Geometry: final body of the model. Coordinates: model frame, mm. Face numbers are marked on the shaded views. Give positions to 0.01 mm unless a question says otherwise; leave off trailing zeros. Write each loop counter-clockwise with the first axis right and the second up, starting at its lowest first coordinate (ties: lowest second). Pieces come first, ordered by that corner, then holes. Notation, with made-up numbers: (65.25, -27.75) -> (106.25, -27.75) arc R22 ccw to (106.25, 6.25) -> close; hole circle Ø7 at (7, -15.75). An arc over 180 degrees is marked (long way). Answer as a JSON object with one key per item and string values.
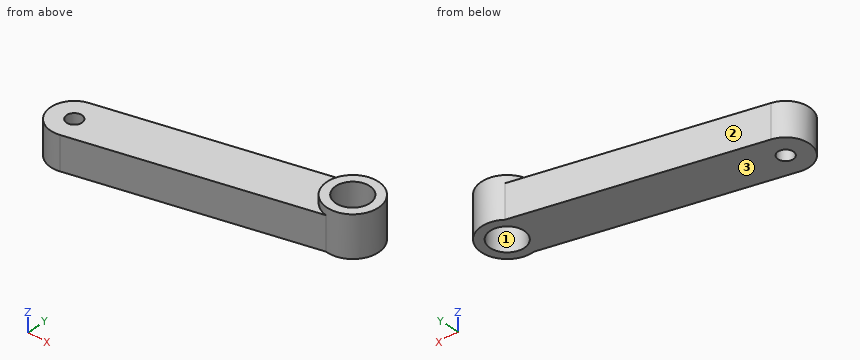
from build123d import *

# Parameters (mm, degrees)
SKETCH3_R           = 4.2545
SKETCH3_R_2         = 1.905
BOSS_EXTRUDE1_DEPTH = 4.191
SKETCH4_R           = 6.436168178
SKETCH4_R_2         = 4.2545
BOSS_EXTRUDE2_DEPTH = 6.096
SKETCH6_R           = 6.436168178
CUT_EXTRUDE1_DEPTH  = 1.905


with BuildPart() as part:
    # Sketch3 → Boss-Extrude1 (new, symmetric)
    with BuildSketch(Plane.XY.offset(6.35)):
        with BuildLine():
            Line((-6.194175956, -60.322809185), (-63.551262793, -74.638203042))
            ThreePointArc((-63.551262793, -74.638203042), (-70.689896022, -70.351217901), (-66.402910881, -63.212584672))
            Line((-66.402910881, -63.212584672), (-9.045824044, -48.897190815))
            ThreePointArc((-9.045824044, -48.897190815), (-1.907190815, -53.184175956), (-6.194175956, -60.322809185))
        make_face()
        with Locations((-7.62, -54.61)):
            Circle(SKETCH3_R, mode=Mode.SUBTRACT)
        with Locations((-64.977086837, -68.925393857)):
            Circle(SKETCH3_R_2, mode=Mode.SUBTRACT)
    extrude(amount=BOSS_EXTRUDE1_DEPTH, both=True)

    # Sketch4 → Boss-Extrude2 (add, symmetric)
    with BuildSketch(Plane.XY.offset(6.35)):
        with Locations((-7.62, -54.61)):
            Circle(SKETCH4_R)
        with Locations((-7.62, -54.61)):
            Circle(SKETCH4_R_2, mode=Mode.SUBTRACT)
    extrude(amount=BOSS_EXTRUDE2_DEPTH, both=True)

    # Sketch6 → Cut-Extrude1 (cut)
    with BuildSketch(Plane(origin=(0, 0, 2.159), x_dir=(-1, 0, 0), z_dir=(0, 0, -1))):
        with Locations(Location((7.62, -54.61, 0), (0, 0, 52.168968889))):
            Circle(SKETCH6_R)
    extrude(amount=CUT_EXTRUDE1_DEPTH, mode=Mode.SUBTRACT)


solid = part.part
Q1. Mould query, pull axis X, two halves, no side actions, for the marked faces 1, 2 and 3. Classes: pulls with the +X half, pulls with the -X half, needs draft (parallel to the pull), parting line crosses it, or undercut.
Values:
{"face 1": "undercut", "face 2": "pulls with the -X half", "face 3": "needs draft"}
Q2. First-contact query: P1, Ø7, axis at x = -7.62, y = -54.61, coming from the +Z side; P2, Ø12, axis at x = -24, y = -61.5, coming from the +Z side; P3, Ø2, axis at y = -60.5, z = 4.5, coming from the +X side. Flat tips, straight axial feed; report the tip coordinate or a pass-through.
Values:
{"P1": "through", "P2": "z = 10.54", "P3": "x = -3.44"}
Q3. Cut plane D-D (y = -60.25). Return the cut outline in (x, z), and give its area (3 significant figures).
Values:
{"outline": "(-54.53, 2.16) -> (-4.52, 2.16) -> (-4.52, 12.45) -> (-10.72, 12.45) -> (-10.72, 10.54) -> (-54.53, 10.54) -> close", "area": "431 mm²"}
Q4. Material intervals for L1, parallel to Y at x = -7.62, z = 5.5; L2, parallel to Z at x = -20, y = -57.5; L3, parallel to Y at x = -41.5, z = 4, sorted ascending. Write a range as from..to.
Values:
{"L1": "-61.05..-58.86, -50.36..-48.17", "L2": "2.16..10.54", "L3": "-69.13..-57"}
Q5. Cut plane C-C (z = 3). Return the cut outline in (x, y) (1 decimal).
Values:
{"outline": "(-66.4, -63.2) arc R5.9 ccw to (-63.6, -74.6) -> (-8.7, -61) arc R6.4 ccw (long way) to (-11.6, -49.5) -> close; hole circle Ø3.8 at (-65, -68.9); hole circle Ø8.5 at (-7.6, -54.6)"}
Q6. Cut plane B-B (y = -54.61). Return the cut outline in (x, z).
Values:
{"outline": "(-31.94, 2.16) -> (-11.87, 2.16) -> (-11.87, 12.45) -> (-14.06, 12.45) -> (-14.06, 10.54) -> (-31.94, 10.54) -> close; (-3.37, 2.16) -> (-1.18, 2.16) -> (-1.18, 12.45) -> (-3.37, 12.45) -> close"}
Q7. Cut plane A-A (x = -7.62). Return the cut outline in (y, z), and give its area (3 significant figures).
Values:
{"outline": "(-61.05, 2.16) -> (-58.86, 2.16) -> (-58.86, 12.45) -> (-61.05, 12.45) -> close; (-50.36, 2.16) -> (-48.17, 2.16) -> (-48.17, 12.45) -> (-50.36, 12.45) -> close", "area": "44.9 mm²"}
